Autodesk Inventor part; units mm, degrees
ref_plane "YZ Plane" through (0, 0, 0) normal (1, 0, 0) x (0, 1, 0)
ref_plane "XZ Plane" through (0, 0, 0) normal (0, 1, 0) x (-1, 0, 0)
ref_plane "XY Plane" through (0, 0, 0) normal (0, 0, 1) x (1, 0, 0)
sketch "스케치1" plane through (0, 0, 0) normal (1, 0, 0) x (0, 1, 0)
  circle A0 centre (0, 0) radius 15
  dimension "d0" = 30
extrude "돌출1" add sketch "스케치1" along normal mid plane 144
sketch "스케치2" plane through (72, 0, 0) normal (1, 0, 0) x (0, 0, -1)
  circle A0 centre (0, 0) radius 5
  dimension "d3" = 10
sketch "스케치3" plane through (-72, 0, 0) normal (-1, 0, 0) x (0, 0, 1)
  circle A0 centre (0, 0) radius 5
  dimension "d4" = 10
extrude "돌출2" add sketch "스케치3" along normal blind 3
extrude "돌출3" add sketch "스케치2" along normal blind 3
sketch "스케치4" plane through (75, 0, 0) normal (1, 0, 0) x (0, 0, -1)
  line L0 (0, 7.5) -> (6.4952, 3.75)
  line L1 (6.4952, 3.75) -> (6.4952, -3.75)
  line L2 (6.4952, -3.75) -> (0, -7.5)
  line L3 (0, -7.5) -> (-6.4952, -3.75)
  line L4 (-6.4952, -3.75) -> (-6.4952, 3.75)
  line L5 (-6.4952, 3.75) -> (0, 7.5)
  point P0 (0, 0)
  point P1 (0, 0)
  dimension "d9" = 15
extrude "돌출4" add sketch "스케치4" along normal blind 5
sketch "스케치5" plane through (-75, 0, 0) normal (-1, 0, 0) x (0, 0, 1)
  circle A0 centre (0, 0) radius 5
  line L0 (0, 7.5) -> (6.4952, 3.75)
  line L1 (6.4952, 3.75) -> (6.4952, -3.75)
  line L2 (6.4952, -3.75) -> (0, -7.5)
  line L3 (0, -7.5) -> (-6.4952, -3.75)
  line L4 (-6.4952, -3.75) -> (-6.4952, 3.75)
  line L5 (-6.4952, 3.75) -> (0, 7.5)
  dimension "d12" = 15
extrude "돌출5" add sketch "스케치5" along normal blind 5 contours A0 | L0 L1 L2 L3 L4 L5
sketch "스케치11" plane through (0, 0, 0) normal (0, 1, 0) x (-1, 0, 0)
  line L0 (72, 5) -> (72, -5)
  line L1 (72, 0) -> (72, 275)
  line L2 (-72, 15) -> (-72, -15)
  line L3 (72, 275) -> (-72, 275)
  line L4 (-72, 275) -> (-72, 0)
  line L5 (72, 0) -> (-72, 0)
  line L6 (-75, 6.4952) -> (-75, 0)
  point P0 (0, 0)
  dimension "d32" = 275
extrude "돌출12" add sketch "스케치11" along normal mid plane 5
sketch "스케치12" plane through (0, 2.5, 0) normal (0, 1, 0) x (1, 0, 0)
  line L0 (-72, -14.7902) -> (72, -14.7902)
  line L1 (-72, -14.7902) -> (-17.5, -275)
  line L2 (-72, -275) -> (72, -275)
  line L3 (0, -275) -> (0, -66.6038)
  line L4 (72, -14.7902) -> (17.5, -275)
  line L5 (-72, -14.7902) -> (-72, -275)
  line L6 (72, -275) -> (72, -14.7902)
  point P0 (0, 0)
  dimension "d37" = 35
extrude "돌출13" cut sketch "스케치12" against normal blind 5 contours L1 L2 L5 | L6 L2 L4
sketch "스케치13" plane through (0, 2.5, 0) normal (0, 1, 0) x (1, 0, 0)
  line L0 (-17.5, -275) -> (17.5, -275)
  circle A0 centre (0, -275) radius 17.5
  point P0 (0, 0)
extrude "돌출14" add sketch "스케치13" against normal blind 5 contours L0 A0 picked at (2.0685, -280.4543)
sketch "스케치14" plane through (0, 2.5, 0) normal (0, 1, 0) x (1, 0, 0)
  arc A0 (-17.5, -275) -> (17.5, -275) centre (0, -275) ccw
  circle A1 centre (0, -275) radius 5
  line L0 (-72, -14.7902) -> (-17.5, -275)
  line L1 (17.5, -275) -> (72, -14.7902)
  line L2 (-72, -14.7902) -> (72, -14.7902)
  line L3 (-72, -14.7902) -> (-17.5, -275)
  arc A2 (-17.5, -275) -> (17.5, -275) centre (0, -275) ccw
  line L4 (47.3771, -34.7902) -> (4.8938, -237.6263)
  line L5 (-4.8938, -237.6263) -> (-47.3771, -34.7902)
  line L6 (-47.3771, -34.7902) -> (47.3771, -34.7902)
  arc A3 (-4.8938, -237.6263) -> (4.8938, -237.6263) centre (0, -236.6013) ccw
  point P0 (0, 0)
  dimension "d40" = 10
  dimension "d41" = 20
  dimension "d42" = 5
extrude "돌출15" cut sketch "스케치14" against normal blind 5 contours A1 | L4 A3 L5 L6
properties part number "link"
Here's how the part is built. I have some questions about the finished solid (model axes, mm). A direction names the side the tool comes from. Give positions to 0.01 mm unless a question says otherwise; leave off trailing zeros. Loops run counter-clockwise (first coordinate to the right, second up) from the corner with the lowest first, then second, coordinate; pieces in that order, holes last. Notation, with made-up numbers: (63, -40) -> (72, -40) arc R10 cw to (72, -24) -> close; hole circle Ø10 at (64.25, -17.75). An arc over 180 degrees is marked (long way). Answer as a JSON object with one key per item and string values. Group by question number.
Item 1: Imagine slicing it at D-D on x = -67. Write out the boundary of the cut face in (y, z), then the cut area to 3 significant figures.
Item 2: Imagine slicing it at C-C on z = 263. Write out the boundary of the cut face in (x, y), then the cut area to 3 significant figures.
Item 3: On a 3-axis mill with a long thin cutter (end or side, diameter ignored), from which of +Z, -Z, +X, -X, +Y, -Y can I reach the whole of each face in a straight line? I mean faces 1 (the flat face through (26.433, 0.035, 134.788)), 2 (the flat face through (26, -2.5, 143)), 3 (the flat face through (-75, 2, -5)), 4 (the flat face through (26, 2.5, 143)). Say none if no direction works.
Item 4: Imagine slicing it at B-B on z = 170.5. Write out the boundary of the cut face in (x, y), then the cut area to 3 significant figures.
Item 5: I need wall thicknesses on L1, parallel to Z at x = 0, y = 1.4; L2, parallel to Z at x = 0, y = -1.1; L3, parallel to X at y = -0.3, z = 275. Which ranges of each line are inside material? Lowest first, please.
Item 6: Will these pins go through, and if not, where does the flat tip stop? pin 1 (2 mm diameter, centred on y = -1.5, z = 155.5, fed in from -X); pin 2 (2.5 mm diameter, centred on x = -8.5, y = 0, fed in from +Z); pin 3 (8 mm diameter, centred on x = 12, z = 186.5, fed in from +Y).
Item 7: Imagine slicing it at A-A on x = 0. Write out the boundary of the cut face in (y, z), then the cut area to 3 significant figures.
Item 8: Thinking about a two-plate mould opening in X: for faces 5 (the flat face through (80, 0, 0)), 6 (the cylindrical face through (-0.385, 0.035, 292.496)), 7 (the cylindrical face through (73.48, 4.88, 1.08)), which applies, pulls with the +X half, pulls with the -X half, needs draft (parallel to the pull), parting line crosses it, or undercut?
Answer list:
{
 "1": {"outline": "(-2.5, 14.79) arc R15 ccw (long way) to (2.5, 14.79) -> (2.5, 38.66) -> (-2.5, 38.66) -> close", "area": "826 mm2"},
 "2": {"outline": "(-20.01, -2.5) -> (20.01, -2.5) -> (20.01, 2.5) -> (-20.01, 2.5) -> close", "area": "200 mm2"},
 "3": {"face 1": "+Y, -Y", "face 2": "+Z, +X, -X, -Y", "face 3": "none", "face 4": "+Z, +X, -X, +Y"},
 "4": {"outline": "(-39.39, -2.5) -> (-18.95, -2.5) -> (-18.95, 2.5) -> (-39.39, 2.5) -> close; (18.95, -2.5) -> (39.39, -2.5) -> (39.39, 2.5) -> (18.95, 2.5) -> close", "area": "204 mm2"},
 "5": {"L1": "z = -14.93 to 34.79, 241.6 to 270, 280 to 292.5", "L2": "z = -14.96 to 34.79, 241.6 to 270, 280 to 292.5", "L3": "x = -17.5 to -5, 5 to 17.5"},
 "6": {"pin 1": "stops at x = -42.74", "pin 2": "stops at z = 290.93", "pin 3": "stops at y = 2.5"},
 "7": {"outline": "(-2.5, 14.79) arc R15 ccw (long way) to (2.5, 14.79) -> (2.5, 34.79) -> (-2.5, 34.79) -> close; (-2.5, 241.6) -> (2.5, 241.6) -> (2.5, 270) -> (-2.5, 270) -> close; (-2.5, 280) -> (2.5, 280) -> (2.5, 292.5) -> (-2.5, 292.5) -> close", "area": "1,010 mm2"},
 "8": {"face 5": "pulls with the +X half", "face 6": "parting line crosses it", "face 7": "undercut"}
}
